Model file for the job. Use its own axes, mm. A direction names the side the tool comes from. Give positions to 0.01 mm unless a question says otherwise; leave off trailing zeros. Order: outer loops, then holes, each group sorted by start corner. A loop starts at its lowest first (then second) coordinate and runs counter-clockwise, first axis right, second up. Notation, with made-up numbers: (-35, -8.75) - (22, -8.75) arc R28 ccw to (22, 26.25) - close; hole circle Ø5 at (57.25, 15.25). An arc over 180 degrees is marked (long way). Return JSON: item names as keys, results as strings. Group by question number.
Autodesk Fusion 360 part; units mm, degrees
sketch "スケッチ1" plane through (0, 0, 0) normal (0, 0, 1) x (1, 0, 0)
  line L0 (-51.75, 40) -> (51.75, 40)
  line L1 (51.75, 40) -> (51.75, -40)
  line L2 (51.75, -40) -> (-51.75, -40)
  line L3 (-51.75, -40) -> (-51.75, 40)
  dimension "d1" = 103.5
  dimension "d2" = 80
  dimension "d32" = 51.75
  dimension "d33" = 40
extrude "押し出し1" add sketch "スケッチ1" along normal blind 2.5 makes body 1
extrude "押し出し4" add sketch "スケッチ1" along normal blind 43 separate body makes body 2
shell "シェル2" thickness 2.5 removed faces 1 at (-17.25, -13.3333, 0) on bodies 2
sketch "スケッチ2" plane through (0, -40, 0) normal (0, -1, 0) x (1, 0, 0)
  line L0 (-51.75, 0) -> (51.75, 0)
  line L1 (51.75, 0) -> (51.75, 43)
  line L2 (51.75, 43) -> (-51.75, 43)
  line L3 (-51.75, 43) -> (-51.75, 0)
  line L4 (-14.5, 0) -> (-14.5, 15.5)
  arc A0 (-1.5, 15.5) -> (-14.5, 15.5) centre (-8, 15.5) ccw
  line L5 (-1.5, 15.5) -> (-1.5, 0)
  line L6 (-14.5, 0) -> (-1.5, 0)
  dimension "d13" = 13
  dimension "d45" = 15.5
  dimension "d46" = 8
extrude "押し出し5" cut sketch "スケッチ2" against normal blind 20 contours L0 L4 A0 L5 L6 bodies 2
sketch "スケッチ3" plane through (0, 40, 0) normal (0, 1, 0) x (-1, 0, 0)
  line L0 (-25, -15) -> (-25, 10)
  arc A0 (-15, 10) -> (-25, 10) centre (-20, 10) ccw
  line L1 (-15, 10) -> (-15, -15)
  line L2 (-15, -15) -> (-25, -15)
  line L3 (-51.75, 0) -> (51.75, 0)
  line L4 (51.75, 0) -> (51.75, 43)
  line L5 (51.75, 43) -> (-51.75, 43)
  line L6 (-51.75, 43) -> (-51.75, 0)
  dimension "d17" = 10
  dimension "d42" = 10
  dimension "d44" = 20
extrude "押し出し6" cut sketch "スケッチ3" against normal blind 16 contours L0 A0 L1 L3 bodies 2
fillet "フィレット1" radius 2 4 edges at (-51.75, 40, 21.5) (51.75, 40, 21.5) (51.75, -40, 21.5) (-51.75, -40, 21.5) 1 faces at (-17.25, -13.3333, 43) on bodies 2
fillet "フィレット1" radius 1.5 6 edges at (-14.5, -40, 7.75) (-8, -40, 22) (-1.5, -40, 7.75) (25, 40, 5) (20, 40, 15) (15, 40, 5) on bodies 2
sketch "スケッチ4" plane through (0, 0, 2.5) normal (0, 0, 1) x (-1, 0, 0)
  line L0 (51.75, 40) -> (-51.75, 40)
  line L1 (-51.75, 40) -> (-51.75, -40)
  line L2 (-51.75, -40) -> (51.75, -40)
  line L3 (51.75, -40) -> (51.75, 40)
  line L4 (47.75, -36) -> (-47.75, -36)
  line L5 (-47.75, -36) -> (-47.75, 36)
  line L6 (-47.75, 36) -> (47.75, 36)
  line L7 (47.75, 36) -> (47.75, -36)
  dimension "d20" = 95.5
  dimension "d21" = 72
  dimension "d22" = 47.75
  dimension "d23" = 36
extrude "押し出し7" add sketch "スケッチ4" along normal blind 2 contours L4 L5 L6 L7 bodies 1
sketch "スケッチ6" plane through (0, 0, 0) normal (0, 0, 1) x (1, 0, 0)
  circle A0 centre (-44.5, -32.75) radius 3
  circle A1 centre (1, -32.75) radius 3
  circle A2 centre (-44.5, 32.75) radius 3
  circle A3 centre (1, 32.75) radius 3
  circle A4 centre (6, -14.75) radius 3
  circle A5 centre (43, -14.75) radius 3
  circle A6 centre (43, 22.75) radius 3
  circle A7 centre (6, 22.75) radius 3
  circle A8 centre (-44.5, -32.75) radius 1.65
  circle A9 centre (1, -32.75) radius 1.65
  circle A10 centre (6, -14.75) radius 1.65
  circle A11 centre (43, -14.75) radius 1.65
  circle A12 centre (43, 22.75) radius 1.65
  circle A13 centre (6, 22.75) radius 1.65
  circle A14 centre (1, 32.75) radius 1.65
  circle A15 centre (-44.5, 32.75) radius 1.65
  dimension "d26" = 6
  dimension "d27" = 45.5
  dimension "d28" = 65.5
  dimension "d29" = 32.75
  dimension "d30" = 37
  dimension "d31" = 37.5
  dimension "d34" = 44.5
  dimension "d35" = 5
  dimension "d39" = 3.3
  dimension "d57" = 10
extrude "押し出し8" cut sketch "スケッチ6" along normal blind 2 contours A0 | A1 | A2 | A3 | A4 | A5 | A6 | A7 | A8 | A9 | A10 | A11 | A12 | A13 | A14 | A15 bodies 1
extrude "押し出し9" cut sketch "スケッチ6" along normal through all contours A8 | A9 | A10 | A11 | A12 | A13 | A14 | A15 bodies 1
sketch "スケッチ8" plane through (0, 0, 2.5) normal (0, 0, 1) x (-1, 0, 0)
  line L0 (-47.75, -36) -> (-47.75, 36)
  line L1 (51.75, 40) -> (-51.75, 40)
  line L2 (-51.75, 40) -> (-51.75, -40)
  line L3 (-51.75, -40) -> (51.75, -40)
  line L4 (-37, -37.25) -> (-49, -25.25)
  line L5 (-49, -37.25) -> (-37, -37.25)
  line L6 (-49, 37.25) -> (-49, 25.25)
  line L7 (-49, 25.25) -> (-37, 37.25)
  line L8 (-37, 37.25) -> (-49, 37.25)
  line L9 (-49, -37.25) -> (-49, -25.25)
  line L10 (49, -25) -> (44, -25)
  line L11 (44, -25) -> (44, 25)
  line L12 (44, 25) -> (49, 25)
  line L13 (49, 25) -> (49, -25)
  line L14 (39.5, -37.25) -> (4.5, -37.25)
  line L15 (4.5, -37.25) -> (4.5, -32.25)
  line L16 (4.5, -32.25) -> (39.5, -32.25)
  line L17 (39.5, -32.25) -> (39.5, -37.25)
  line L18 (4.5, 32.25) -> (39.5, 32.25)
  line L19 (39.5, 32.25) -> (39.5, 37.25)
  line L20 (39.5, 37.25) -> (4.5, 37.25)
  line L21 (4.5, 37.25) -> (4.5, 32.25)
  dimension "d50" = 49
  dimension "d51" = 74.5
  dimension "d52" = 37.25
  dimension "d53" = 12
  dimension "d58" = 50
  dimension "d59" = 5
  dimension "d60" = 49
  dimension "d61" = 25
  dimension "d63" = 35
  dimension "d64" = 4.5
extrude "押し出し10" add sketch "スケッチ8" along normal blind 5 bodies 1
fillet "フィレット2" radius 2 4 edges at (-51.75, -40, 1.25) (51.75, -40, 1.25) (51.75, 40, 1.25) (-51.75, 40, 1.25) on bodies 1
sketch "スケッチ10" plane through (0, 0, 43) normal (0, 0, 1) x (-1, 0, 0)
  line L0 (49.75, 38) -> (-49.75, 38)
  line L1 (-49.75, 38) -> (-49.75, -38)
  line L2 (-49.75, -38) -> (49.75, -38)
  line L3 (49.75, -38) -> (49.75, 38)
  line L4 (38, -15) -> (18, -15)
  line L5 (18, -15) -> (18, 20)
  line L6 (18, 20) -> (38, 20)
  line L7 (38, 20) -> (38, -15)
  dimension "d73" = 15
  dimension "d74" = 20
  dimension "d75" = 18
  dimension "d76" = 20
extrude "押し出し13" cut sketch "スケッチ10" against normal blind 25 contours L4 L5 L6 L7 bodies 2
sketch "スケッチ9" plane through (51.75, 0, 0) normal (1, 0, 0) x (0, 1, 0)
  line L0 (-38, 41) -> (-38, 0)
  line L1 (-38, 0) -> (38, 0)
  line L2 (38, 0) -> (38, 41)
  line L3 (38, 41) -> (-38, 41)
  line L4 (-15, 36) -> (15, 36)
  line L5 (15, 36) -> (15, 33)
  line L6 (15, 33) -> (-15, 33)
  line L7 (-15, 33) -> (-15, 36)
  line L8 (15, 27) -> (-15, 27)
  line L9 (-15, 30) -> (15, 30)
  line L10 (15, 30) -> (15, 27)
  line L11 (-15, 27) -> (-15, 30)
  line L12 (15, 21) -> (-15, 21)
  line L13 (-15, 24) -> (15, 24)
  line L14 (15, 24) -> (15, 21)
  line L15 (-15, 21) -> (-15, 24)
  line L16 (15, 15) -> (-15, 15)
  line L17 (-15, 18) -> (15, 18)
  line L18 (15, 18) -> (15, 15)
  line L19 (-15, 15) -> (-15, 18)
  line L20 (15, 9) -> (-15, 9)
  line L21 (-15, 12) -> (15, 12)
  line L22 (15, 12) -> (15, 9)
  line L23 (-15, 9) -> (-15, 12)
  line L24 (15, 3) -> (-15, 3)
  line L25 (-15, 6) -> (15, 6)
  line L26 (15, 6) -> (15, 3)
  line L27 (-15, 3) -> (-15, 6)
  dimension "d80" = 30
  dimension "d81" = 3
  dimension "d82" = 15
  dimension "d85" = 0
  dimension "d86" = -6
  dimension "d89" = 36
extrude "押し出し14" cut sketch "スケッチ9" against normal blind 10 contours L4 L5 L6 L7 | L8 L9 L10 L11 | L12 L13 L14 L15 | L16 L17 L18 L19 | L20 L21 L22 L23 | L24 L25 L26 L27 bodies 2
sketch "スケッチ11" plane through (0, 0, 43) normal (0, 0, 1) x (-1, 0, 0)
  line L0 (18, -15) -> (18, 20)
  line L1 (18, 20) -> (38, 20)
  line L2 (38, 20) -> (38, -15)
  line L3 (38, -15) -> (18, -15)
  line L4 (49.75, 38) -> (-49.75, 38)
  line L5 (-49.75, 38) -> (-49.75, -38)
  line L6 (-49.75, -38) -> (49.75, -38)
  line L7 (49.75, -38) -> (49.75, 38)
  line L8 (-47, -15) -> (-44, -15)
  line L9 (-44, -15) -> (-44, 15)
  line L10 (-44, 15) -> (-47, 15)
  line L11 (-47, 15) -> (-47, -15)
  line L12 (-41, -15) -> (-38, -15)
  line L13 (-38, -15) -> (-38, 15)
  line L14 (-38, 15) -> (-41, 15)
  line L15 (-41, 15) -> (-41, -15)
  line L16 (-35, -15) -> (-32, -15)
  line L17 (-32, -15) -> (-32, 15)
  line L18 (-32, 15) -> (-35, 15)
  line L19 (-35, 15) -> (-35, -15)
  dimension "d90" = 3
  dimension "d91" = 30
  dimension "d92" = 15
extrude "押し出し15" cut sketch "スケッチ11" against normal blind 20 contours L8 L9 L10 L11 | L12 L13 L14 L15 | L16 L17 L18 L19 bodies 2
hidden bodies 1
equation "d1 = 93.5 mm + 10 mm"
equation "d22 = ( 95.5 / 2 ) * 1 mm"
equation "d28 = 70 mm - 4.5 mm"
equation "d29 = ( 65.5 / 2 ) * 1 mm"
equation "d30 = 43.5 mm - 6.5 mm"
equation "d32 = ( 103.5 / 2 ) * 1 mm"
(1) Drop flat-ended pins along their axis: pin 1 Ø1.2 at (y, z) = (3, 42) entering from +X; pin 2 Ø1.2 at (x, z) = (50.5, 17) entering from -Y; pin 3 Ø1.2 at (x, y) = (51, -2) entering from +Z. Give the stop position or say it passes through.
(2) 3-axis set-ups, long thin cutter, end or side, ignore diameter. For faces 4 (the face through (51, 15, 35)), 5 (the face through (-8, -38, 22)), 6 (the face through (32, 0, 42)), 7 (the face through (20, 38, 15)), 8 (the face through (-1, 37.5, 20)): which of +Z, -Z, +X, -X, +Y, -Y reach the whole face in a straight line?
(3) Pull direction Z, two halves, no side cores. Call faces 1 (the face through (-1, 1, 40.5)), 2 (the face through (-51.75, -1, 20)), 3 (the face through (51, 15, 23)): released by +Z, released by -Z, zero draft, split by the parting line, or undercut.
(4) Slice it at A-A (x = 20). Give the cut face in (y, z).
(5) Slice it at D-D (x = -45). Give the cut face in (y, z), and give its area (3 significant figures).
(6) Slice it at C-C (y = 28). Give the cut face in (x, z), and give its area (3 significant figures).
(7) Drill centre lines: L1, parallel to Y at x = -36.5, z = 23; L2, parallel to X at y = -32, z = 35; L3, parallel to Z at x = 36, y = 7.5. Where is each one in solid material? Low to high.
(8) Slice it at B-B (z = 38). Give the cut face in (x, y), and give its area (3 significant figures).
Result set:
{
 "1": {"pin 1": "stops at x = 51.71", "pin 2": "stops at y = -39.99", "pin 3": "stops at z = 42.89"},
 "2": {"face 4": "+X", "face 5": "-Z, -Y", "face 6": "+Z, -Z", "face 7": "-Z, +Y", "face 8": "-Z"},
 "3": {"face 1": "released by -Z", "face 2": "zero draft", "face 3": "undercut"},
 "4": {"outline": "(-40, 0) - (-37.5, 0) - (-37.5, 40.5) - (37.5, 40.5) - (37.5, 15) - (38.5, 15) arc R1.5 ccw to (40, 16.5) - (40, 41) arc R2 ccw to (38, 43) - (-38, 43) arc R2 ccw to (-40, 41) - close"},
 "5": {"outline": "(-40, 0) - (-37.5, 0) - (-37.5, 40.5) - (37.5, 40.5) - (37.5, 0) - (40, 0) - (40, 41) arc R2 ccw to (38, 43) - (-38, 43) arc R2 ccw to (-40, 41) - close", "area": "401 mm²"},
 "6": {"outline": "(-51.75, 0) - (-49.25, 0) - (-49.25, 40.5) - (49.25, 40.5) - (49.25, 0) - (51.75, 0) - (51.75, 41) arc R2 ccw to (49.75, 43) - (-49.75, 43) arc R2 ccw to (-51.75, 41) - close", "area": "460 mm²"},
 "7": {"L1": "y = -40 to -37.5, 37.5 to 40", "L2": "x = -51.75 to -49.25, 49.25 to 51.75", "L3": "z = 40.5 to 43"},
 "8": {"outline": "(-51.75, -38) arc R2 ccw to (-49.75, -40) - (49.75, -40) arc R2 ccw to (51.75, -38) - (51.75, 38) arc R2 ccw to (49.75, 40) - (-49.75, 40) arc R2 ccw to (-51.75, 38) - close; hole (-49.25, -37.5) - (49.25, -37.5) - (49.25, 37.5) - (-49.25, 37.5) - close", "area": "889 mm²"}
}
